```python
from build123d import *

# Parameters (mm, degrees)
F0_W           = 127
F0_H           = 76.2
F1_DEPTH       = 50.8
F3_D           = 12.7
F3_DEPTH       = 50.8
F3_CBORE_D     = 19.05
F3_CBORE_DEPTH = 12.7
F3_TIP         = 3.8154649308
F5_D           = 12.7
F5_CSINK_D     = 25.4
F5_CSINK_ANGLE = 82
F7_D           = 12.7
F9_D           = 6.35
F9_DEPTH       = 25.4
F9_CBORE_D     = 9.525
F9_CBORE_DEPTH = 6.35
F9_TIP         = 1.9077324654


with BuildPart() as f1:
    # F0 (on Front) → F1 (new body)
    with BuildSketch(Plane.XZ):
        with Locations((2.8626964785, 38.1)):
            Rectangle(F0_W, F0_H)
    extrude(amount=F1_DEPTH)

    # F3
    with Locations(Plane.XY.offset(76.2)):
        with Locations((-41.5873035215, -25.4)):
            CounterBoreHole(F3_D / 2, F3_CBORE_D / 2, F3_CBORE_DEPTH, depth=F3_DEPTH)
            with Locations((0, 0, -(F3_DEPTH + F3_TIP / 2))):  # 118° drill point
                Cone(0, F3_D / 2, F3_TIP, mode=Mode.SUBTRACT)

    # F5 (through all)
    with Locations(Plane.XY.offset(76.2)):
        with Locations((-16.1873035215, -25.4)):
            CounterSinkHole(F5_D / 2, F5_CSINK_D / 2, counter_sink_angle=F5_CSINK_ANGLE)

    # F7 (through all)
    with Locations(Plane.XY.offset(76.2)):
        with Locations((15.5626964785, -25.4)):
            Hole(F7_D / 2)

    # F9
    with Locations(Plane.XY.offset(76.2)):
        with Locations((47.3126964785, -25.4)):
            CounterBoreHole(F9_D / 2, F9_CBORE_D / 2, F9_CBORE_DEPTH, depth=F9_DEPTH)
            with Locations((0, 0, -(F9_DEPTH + F9_TIP / 2))):  # 118° drill point
                Cone(0, F9_D / 2, F9_TIP, mode=Mode.SUBTRACT)


solid = f1.part
```
Input: part model. Units: mm. Frame: model coordinates. A direction names the side the tool comes from. Round coordinates to 2 decimals unless told otherwise and drop trailing zeros. Order: outer loops, then holes, each group sorted by start corner. A loop starts at its lowest first (then second) coordinate and runs counter-clockwise, first axis right, second up. Notation, with made-up numbers: (16.5, 56.5) - (29.5, 56.5) arc R21 cw to (29.5, 89.5) - close; hole circle Ø8 at (0.5, 16.5). An arc over 180 degrees is marked (long way). Answer in a Markdown table with one row per item.
Item 1: Section query B-B (z = 55). Return the cut outline in (x, y) (3 decimals).
Model answer:
| item | result |
|---|---|
| outline | (-60.637, -50.8) - (66.363, -50.8) - (66.363, 0) - (-60.637, 0) - close; hole circle Ø12.7 at (-41.587, -25.4); hole circle Ø12.7 at (-16.187, -25.4); hole circle Ø12.7 at (15.563, -25.4); hole circle Ø6.35 at (47.313, -25.4) |
Item 2: Section query C-C (z = 47). Return the cut outline in (x, y), then the cut area to 3 significant figures.
Model answer:
| item | result |
|---|---|
| outline | (-60.64, -50.8) - (66.36, -50.8) - (66.36, 0) - (-60.64, 0) - close; hole circle Ø12.7 at (-41.59, -25.4); hole circle Ø12.7 at (-16.19, -25.4); hole circle Ø12.7 at (15.56, -25.4) |
| area | 6,070 mm² |
Item 3: Mould query, pull axis Y, two halves, no side actions, for faces 1 (the flat face through (66.363, -25, 38)), 2 (the flat face through (2, 0, 39)), 3 (the flat face through (-40, -32, 63.5)). Classes: released by +Y, released by -Y, zero draft, split by the parting line, or undercut.
Model answer:
| item | result |
|---|---|
| face 1 | zero draft |
| face 2 | released by +Y |
| face 3 | undercut |
Item 4: Section query D-D (z = 15). Return the cut outline in (x, y).
Model answer:
| item | result |
|---|---|
| outline | (-60.64, -50.8) - (66.36, -50.8) - (66.36, 0) - (-60.64, 0) - close; hole circle Ø12.7 at (-16.19, -25.4); hole circle Ø12.7 at (15.56, -25.4) |
Item 5: Reachability of faces 4 (the cylindrical face through (-36.548, -29.264, 44.183)), 5 (the flat face through (2, -50.8, 39)) from +Z, -Z, +X, -X, +Y, -Y: full face, straight path, thin tool, end or side. Return the list, or none.
Model answer:
| item | result |
|---|---|
| face 4 | +Z |
| face 5 | +Z, -Z, +X, -X, -Y |
Item 6: Section query A-A (x = 19). Return the cut outline in (y, z).
Model answer:
| item | result |
|---|---|
| outline | (-50.8, 0) - (-30.74, 0) - (-30.74, 76.2) - (-50.8, 76.2) - close; (-20.06, 0) - (0, 0) - (0, 76.2) - (-20.06, 76.2) - close |
Item 7: Line query: line 1 (X direction, y = -25, z = 45); line 2 (X direction, y = -25, z = 73); line 3 (X direction, y = -30, z = 7.5). Output: solid intervals per line, ascending.
Model answer:
| item | result |
|---|---|
| line 1 | x = -60.64 to -47.92, -35.25 to -22.52, -9.85 to 9.23, 21.9 to 66.36 |
| line 2 | x = -60.64 to -51.1, -32.07 to -26.1, -6.28 to 9.23, 21.9 to 42.57, 52.06 to 66.36 |
| line 3 | x = -60.64 to -20.56, -11.81 to 11.19, 19.94 to 66.36 |
Item 8: Pin query (flat end, axial travel): pin 1 (7.5 mm diameter, centred on x = 47.31, y = -25.4, fed in from +Z); pin 2 (11.5 mm diameter, centred on x = -16.19, y = -25.4, fed in from -Z); pin 3 (5.5 mm diameter, centred on x = -40.5, y = -25.5, fed in from +Z). Return the tip coordinate at first contact, or that it passes through.
Model answer:
| item | result |
|---|---|
| pin 1 | stops at z = 69.85 |
| pin 2 | passes through |
| pin 3 | stops at z = 23.89 |
